from build123d import *

# Parameters (mm, degrees)
ESQUISSE1_W             = 50.8
ESQUISSE1_H             = 82.55
BOSS_EXTRU_1_DEPTH      = 6.35
ESQUISSE2_W             = 50.8
ESQUISSE2_H             = 82.55
BOSS_EXTRU_2_DEPTH      = 6.35
ESQUISSE4_R             = 1.778
ESQUISSE4_R_2           = 1.651
BOSS_EXTRU_3_DEPTH      = 6.35
ESQUISSE5_W             = 38.1
ESQUISSE5_H             = 38.1
ENL_V_MAT_EXTRU_1_DEPTH = 6.35
ESQUISSE7_W             = 33.02
ESQUISSE7_H             = 44.45
ENL_V_MAT_EXTRU_2_DEPTH = 6.35
BOSS_EXTRU_4_DEPTH      = 8.89
CONG_1_R                = 6.35


with BuildPart() as part:
    # Esquisse1 → Boss.-Extru.1 (new body)
    with BuildSketch(Plane.XY):
        Rectangle(ESQUISSE1_W, ESQUISSE1_H)
    extrude(amount=BOSS_EXTRU_1_DEPTH)

    # Esquisse2 → Boss.-Extru.2 (add)
    with BuildSketch(Plane(origin=(0, 41.275, 0), x_dir=(1, 0, 0), z_dir=(0, 1, 0))):
        with Locations((0, -47.625)):
            Rectangle(ESQUISSE2_W, ESQUISSE2_H)
    extrude(amount=-BOSS_EXTRU_2_DEPTH)

    # Esquisse4 → Boss.-Extru.3 (add)
    with BuildSketch(Plane.ZY.offset(25.4)):
        Polygon((6.35, -32.426920908), (31.045704333, -7.731216575), (6.35, 16.964487758), (6.35, 25.944743879), (35.535832393, -3.241088515), (44.516088515, 5.739167607), (15.330256121, 34.925), (24.310512242, 34.925), (49.006216575, 10.229295667), (73.701920908, 34.925), (82.682177029, 34.925), (6.35, -41.407177029), align=None)
        with Locations(Location((28.082219813, -15.184829156, 0), (0, 0, 270))):
            Circle(ESQUISSE4_R, mode=Mode.SUBTRACT)
        with Locations(Location((69.211792847, 25.944743879, 0), (0, 0, 270))):
            Circle(ESQUISSE4_R_2, mode=Mode.SUBTRACT)
    boss_extru_3 = extrude(amount=-BOSS_EXTRU_3_DEPTH)

    # Symétrie1: Boss.-Extru.3 across plane
    add(boss_extru_3.mirror(Plane(origin=(0, 0, 0), x_dir=(0, 0, 1), z_dir=(1, 0, 0))))

    # Esquisse5 → Enlèv. mat.-Extru.1 (cut)
    with BuildSketch(Plane(origin=(0, 41.275, 0), x_dir=(1, 0, 0), z_dir=(0, 1, 0))):
        with Locations((0, -60.96)):
            Rectangle(ESQUISSE5_W, ESQUISSE5_H)
    extrude(amount=-ENL_V_MAT_EXTRU_1_DEPTH, mode=Mode.SUBTRACT)

    # Esquisse7 → Enlèv. mat.-Extru.2 (cut)
    with BuildSketch(Plane(origin=(0, 0, 0), x_dir=(-1, 0, 0), z_dir=(0, 0, -1))):
        with Locations((0, -19.05)):
            Rectangle(ESQUISSE7_W, ESQUISSE7_H)
    extrude(amount=-ENL_V_MAT_EXTRU_2_DEPTH, mode=Mode.SUBTRACT)

    # Esquisse8 → Boss.-Extru.4 (add)
    with BuildSketch(Plane(origin=(25.4, 0, 0), x_dir=(0, 0, -1), z_dir=(1, 0, 0))):
        Polygon((0, -41.275), (12.7, -9.525), (0, -9.525), align=None)
    boss_extru_4 = extrude(amount=-BOSS_EXTRU_4_DEPTH)

    # Symétrie2: Boss.-Extru.4 across plane
    add(boss_extru_4.mirror(Plane(origin=(0, 0, 0), x_dir=(0, 0, 1), z_dir=(1, 0, 0))))

    # Congé1
    cong_1_edges = [part.edges().sort_by_distance(p)[0] for p in [
        (0, 34.925, 6.35),
        (-22.225, -32.426920908, 6.35),
        (-22.225, -7.731216575, 31.045704333),
        (-22.225, 16.964487758, 6.35),
        (-22.225, 25.944743879, 6.35),
        (-22.225, -3.241088515, 35.535832393),
        (-22.225, 5.739167607, 44.516088515),
        (-22.225, 34.925, 15.330256121),
        (-22.225, 34.925, 24.310512242),
        (-22.225, 10.229295667, 49.006216575),
        (-22.225, 34.925, 73.701920908),
        (-22.225, 34.925, 82.682177029),
        (22.225, -32.426920908, 6.35),
        (22.225, 34.925, 82.682177029),
        (22.225, 34.925, 73.701920908),
        (22.225, 10.229295667, 49.006216575),
        (22.225, 34.925, 24.310512242),
        (22.225, 34.925, 15.330256121),
        (22.225, 5.739167607, 44.516088515),
        (22.225, -3.241088515, 35.535832393),
        (22.225, 25.944743879, 6.35),
        (22.225, 16.964487758, 6.35),
        (22.225, -7.731216575, 31.045704333),
    ]]
    fillet(cong_1_edges, radius=CONG_1_R - 0.0001)  # a hair under: the kernel refuses the full size


solid = part.part
Model file for the job. Use its own axes, mm. A direction names the side the tool comes from. Coordinates: 2 decimals unless noted, no trailing zeros. Write each loop counter-clockwise with the first axis right and the second up, starting at its lowest first coordinate (ties: lowest second). Pieces come first, ordered by that corner, then holes. Notation, with made-up numbers: (-30, 83) - (-2, 83) arc R34 ccw to (-2, 120) - close; hole circle Ø9 at (26, 59.25). An arc over 180 degrees is marked (long way). Write each question's results on one line, items separated by ' | '. Start each with the question number.
1) Cut at D-D (x = 22). Count the separate pieces of the cut face and the enclosed holes in it, then the cut area to 3 significant figures.
2) Cut at A-A (x = 9). Write the cut outline in (y, z) (3 decimals), then the cut area to 3 significant figures.
3) Flat gauge pins, fed straight in: P1, Ø2.5, axis at x = 23, z = -8.5, coming from the +Y side (3 decimals); P2, Ø15, axis at y = -27, z = -8, coming from the +X side; P3, Ø1.9, axis at x = -3.5, z = 2.5, coming from the -Y side (3 decimals); P4, Ø3, axis at x = -19, z = 72, coming from the -Y side. Where does each tip first touch, or does it go through?
4) Cut at C-C (z = 20). Write the cut outline in (x, y) (3 decimals).
5) 3-axis set-ups, long thin cutter, end or side, ignore diameter. For faces 4 (the face through (19.05, 12, 43)), 5 (the face through (-22.269, 21.487, 28.768)), 6 (the face through (0, 38, 41.91)), 7 (the face through (-21.02, -25.62, -6.26)): which of +Z, -Z, +X, -X, +Y, -Y reach the whole face in a straight line?
6) Mould opens along Y. For faces 1 (the face through (-22.27, -3.65, 44.11)), 2 (the face through (22.269, 21.487, 28.768)), 3 (the face through (0, 16, 0)) say: pulls with the +Y half, pulls with the -Y half, needs draft (parallel to the pull), parting line crosses it, or undercut.
7) Cut at B-B (y = 22). Write the cut outline in (x, z).
8) Probe line 1 along X through (y, z) = (-17.5, 4.5); line 2 along X through (y, z) = (22.5, 8); line 3 along Z through (x, y) = (-9, 36). List the from-to ranges inside material, lowest first. Write a range as from..to.
Returned:
1) separate pieces: 1 | enclosed holes: 5 | area: 2,610 mm^2
2) outline: (3.175, 0) - (41.275, 0) - (41.275, 41.91) - (34.925, 41.91) - (34.925, 12.7) arc R6.35 cw to (28.575, 6.35) - (3.175, 6.35) - close; (34.925, 80.01) - (41.275, 80.01) - (41.275, 88.9) - (34.925, 88.9) - close | area: 533 mm^2
3) P1: y = -9.525 | P2: x = 25.4 | P3: y = 3.175 | P4: y = 22.74
4) outline: (-25.4, -27.757) - (-19.05, -27.757) - (-19.05, -18.777) - (-25.4, -18.777) - close; (-25.4, 3.314) - (-19.05, 3.314) - (-19.05, 12.295) - (-25.4, 12.295) - close; (-25.4, 30.255) - (-19.05, 30.255) - (-19.05, 34.925) - (19.05, 34.925) - (19.05, 30.255) - (25.4, 30.255) - (25.4, 41.275) - (-25.4, 41.275) - close; (19.05, -27.757) - (25.4, -27.757) - (25.4, -18.777) - (19.05, -18.777) - close; (19.05, 3.314) - (25.4, 3.314) - (25.4, 12.295) - (19.05, 12.295) - close
5) face 4: -Y | face 5: +X, -X | face 6: +Y, -Y | face 7: -Z, +X, -X, -Y
6) face 1: pulls with the -Y half | face 2: undercut | face 3: needs draft
7) outline: (-25.4, 0) - (25.4, 0) - (25.4, 10.29) - (19.05, 10.29) - (19.05, 6.35) - (-19.05, 6.35) - (-19.05, 10.29) - (-25.4, 10.29) - close; (-25.4, 28.26) - (-19.05, 28.26) - (-19.05, 37.24) - (-25.4, 37.24) - close; (-25.4, 60.78) - (-19.05, 60.78) - (-19.05, 69.76) - (-25.4, 69.76) - close; (19.05, 28.26) - (25.4, 28.26) - (25.4, 37.24) - (19.05, 37.24) - close; (19.05, 60.78) - (25.4, 60.78) - (25.4, 69.76) - (19.05, 69.76) - close
8) line 1: -25.4..-16.51, 16.51..25.4 | line 2: -25.4..-19.05, 19.05..25.4 | line 3: 0..41.91, 80.01..88.9
